```python
from build123d import *

# Parameters (mm, degrees)
BOSS_EXTRUDE1_DEPTH     = 76.2
BOSS_EXTRUDE8_DEPTH     = 6.35
LPATTERN3_COUNT         = 2
LPATTERN3_PITCH         = 69.85
FILLET2_R               = 50.8
SKETCH12_W              = 64.895089707
SKETCH12_H              = 101.6
BOSS_EXTRUDE10_DEPTH    = 4.318
TOP_CIRCLE_CUT_REACH    = 278.774
SKETCH10_R              = 24.13
CUT_EXTRUDE2_DEPTH      = 26.4
CUT_EXTRUDE2_DEPTH_BACK = 98.777385928
FILLET3_R               = 2.54


with BuildPart() as part:
    # Sketch1 → Boss-Extrude1 (new body)
    with BuildSketch(Plane.XY):
        Polygon((0, 0), (0, 342.9), (-34.18639432, 391.723230906), (-30.558898383, 394.263230906), (-23.731659882, 384.51292385), (5.406023084, 342.9), (5.406023084, 0), align=None)
    extrude(amount=BOSS_EXTRUDE1_DEPTH)

    # Sketch9 → Boss-Extrude8 (add)
    with BuildSketch(Plane.XY):
        Polygon((5.406023084, 0), (30.806023084, 0), (30.806023084, 342.9), (-5.158898383, 394.263230906), (-30.558898383, 394.263230906), (5.406023084, 342.9), align=None)
    boss_extrude8 = extrude(amount=BOSS_EXTRUDE8_DEPTH)

    # LPattern3: Boss-Extrude8 ×2
    with Locations(*[(0, 0, i * LPATTERN3_PITCH) for i in range(1, LPATTERN3_COUNT)]):
        add(boss_extrude8)

    # Fillet2
    fillet2_edges = [part.edges().sort_by_distance(p)[0] for p in [
        (0, 342.9, 38.1),
        (30.806023084, 342.9, 3.175),
        (5.406023084, 342.9, 38.1),
        (30.806023084, 342.9, 73.025),
    ]]
    fillet(fillet2_edges, radius=FILLET2_R)

    # Sketch12 → Boss-Extrude10 (add)
    with BuildSketch(Plane(origin=(164.737795771, 115.350646427, 0), x_dir=(0, 0, -1), z_dir=(0.819152044, 0.573576436, 0))):
        with Locations((-37.402455147, 391.289395618)):
            Rectangle(SKETCH12_W, SKETCH12_H)
    extrude(amount=-BOSS_EXTRUDE10_DEPTH)

    # Sketch10 → Top Circle Cut (cut, up to next)
    with BuildSketch(Plane(origin=(164.737795771, 115.350646427, 0), x_dir=(0, 0, -1), z_dir=(0.819152044, 0.573576436, 0)), mode=Mode.PRIVATE) as top_circle_cut_sk1:
        with Locations((-38.1, 383.669395618)):
            Circle(SKETCH10_R)
    top_circle_cut_tool1 = extrude(top_circle_cut_sk1.sketch, amount=-TOP_CIRCLE_CUT_REACH, mode=Mode.PRIVATE) & part.part
    add(top_circle_cut_tool1.solids().sort_by_distance((-55.325929, 429.634216, 38.1))[0], mode=Mode.SUBTRACT)

    # Sketch13 → Cut-Extrude2 (cut, two sides)
    with BuildSketch(Plane(origin=(5.406023084, 0, 0), x_dir=(0, 0, -1), z_dir=(1, 0, 0))) as cut_extrude2_sk:
        Polygon((-38.1, 31.75), (-69.85, 0), (-6.35, 0), align=None)
    extrude(amount=CUT_EXTRUDE2_DEPTH, mode=Mode.SUBTRACT)
    extrude(cut_extrude2_sk.sketch, amount=-CUT_EXTRUDE2_DEPTH_BACK, mode=Mode.SUBTRACT)

    # Fillet3
    fillet3_edges = [part.edges().sort_by_distance(p)[0] for p in [
        (2.703011542, 31.75, 38.1),
    ]]
    fillet(fillet3_edges, radius=FILLET3_R)


solid = part.part
```
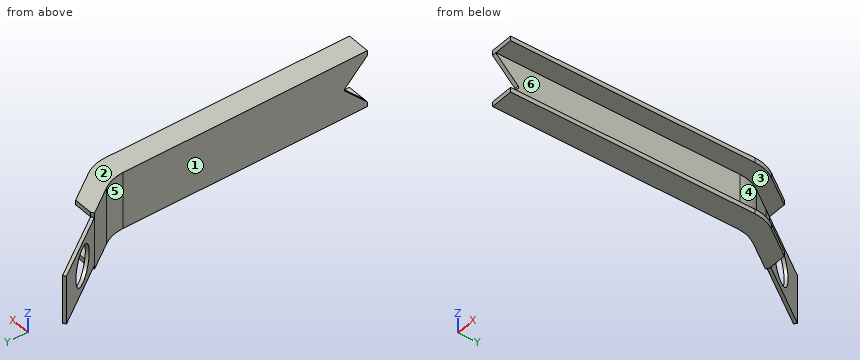
Check sheet for the modelled part. Datum: model origin and axes. Units: mm. Face numbers are marked on the shaded views. A direction names the side the tool comes from. Give positions to 0.01 mm unless a question says otherwise; leave off trailing zeros. Order: outer loops, then holes, each group sorted by start corner. A loop starts at its lowest first (then second) coordinate and runs counter-clockwise, first axis right, second up. Notation, with made-up numbers: (17.5, 48) -> (42.5, 48) arc R7 ccw to (42.5, 55) -> close; hole circle Ø6 at (13.5, 79). An arc over 180 degrees is marked (long way). Use CSV: the item, a comma, the result in double quotes. Start each with the question number.
1) Material ranges on line 1 (Z direction, x = 9, y = 82); line 2 (X direction, y = 108.5, z = 24); line 3 (X direction, y = 132.5, z = 71), recorded low to high. Write a range as from..to.
2) Mould release check, pull along Z, two halves, no side actions. Record for the marked faces 1, 2 and 3: released by +Z, released by -Z, zero draft, split by the parting line, or undercut.
3) Go/stop test with flat-tipped pins: P1, Ø10, axis at y = 114.5, z = 33, coming from the -X side; P2, Ø1.5, axis at y = 395, z = 22, coming from the +X side; P3, Ø6, axis at x = 6.5, z = 16.5, coming from the -Y side; P4, Ø18.5, axis at x = 14.5, y = 202, coming from the -Z side. Record where each tip stops, or that it passes through.
4) Sectioned sample at A-A, the plane y = 66. Record the boundary of the cut face in (x, z), plus the area to 3 significant figures.
5) Sectioned sample at C-C, the plane x = -78. Record the boundary of the cut face in (y, z), plus the area to 3 significant figures.
6) Sectioned sample at B-B, the plane z = 46.5. Record the boundary of the cut face in (x, y).
7) Set-up check for the marked faces 4, 5 and 6: record each of +Z, -Z, +X, -X, +Y, -Y from which the full face is reachable in a straight line by a thin tool's end or side.
Recorded:
1,line 1,"0..6.35, 69.85..76.2"
1,line 2,"0..5.41"
1,line 3,"0..30.81"
2,face 1,"zero draft"
2,face 2,"released by +Z"
2,face 3,"undercut"
3,P1,"x = 0"
3,P2,"x = -30.55"
3,P3,"y = 7.36"
3,P4,"z = 0"
4,outline,"(0, 0) -> (30.81, 0) -> (30.81, 6.35) -> (5.41, 6.35) -> (5.41, 69.85) -> (30.81, 69.85) -> (30.81, 76.2) -> (0, 76.2) -> close"
4,area,"735 mm2"
5,outline,"(454.49, 4.95) -> (462.02, 4.95) -> (462.02, 69.85) -> (454.49, 69.85) -> close"
5,area,"489 mm2"
6,outline,"(-92.37, 475.01) -> (-71.84, 445.69) -> (-68.3, 448.16) -> (-88.83, 477.49) -> close; (-45.89, 408.63) -> (-34.1, 391.79) -> (-34.19, 391.72) -> (-9.19, 356.02) arc R50.8 cw to (0, 326.88) -> (0, 23.35) -> (5.41, 23.35) -> (5.41, 326.88) arc R50.8 ccw to (-3.78, 356.02) -> (-42.35, 411.1) -> close"
7,face 4,"+X, +Y"
7,face 5,"+Z, -Z, -X, -Y"
7,face 6,"+X, +Y, -Y"
